Could you check a few things on this model? Use its own coordinates, in mm. A direction names the side the tool comes from. Round coordinates to 2 decimals unless told otherwise and drop trailing zeros. Loops run counter-clockwise (first coordinate to the right, second up) from the corner with the lowest first, then second, coordinate; pieces in that order, holes last. Notation, with made-up numbers: (71, -10) -> (124, -10) arc R18 ccw to (124, 10) -> close; hole circle Ø8 at (-40, -31). An arc over 180 degrees is marked (long way). One line per item, written item: value.
Autodesk Inventor part; units mm, degrees
ref_plane "YZ Plane" through (0, 0, 0) normal (1, 0, 0) x (0, 1, 0)
ref_plane "XZ Plane" through (0, 0, 0) normal (0, 1, 0) x (-1, 0, 0)
ref_plane "XY Plane" through (0, 0, 0) normal (0, 0, 1) x (1, 0, 0)
sketch "Sketch1" plane through (0, 0, 0) normal (0, 0, 1) x (1, 0, 0)
  line L0 (7.62, 0) -> (72.898, 0)
  line L1 (0, 7.62) -> (0, 31.242)
  line L2 (7.62, 38.862) -> (72.898, 38.862)
  line L3 (80.518, 31.242) -> (80.518, 7.62)
  arc A0 (7.62, 38.862) -> (0, 31.242) centre (7.62, 31.242) ccw
  arc A1 (80.518, 31.242) -> (72.898, 38.862) centre (72.898, 31.242) ccw
  arc A2 (72.898, 0) -> (80.518, 7.62) centre (72.898, 7.62) ccw
  arc A3 (0, 7.62) -> (7.62, 0) centre (7.62, 7.62) ccw
  point P0 (0, 0)
  point P1 (80.518, 0)
  point P2 (0, 38.862)
  dimension "d2" = 80.518
  dimension "d3" = 38.862
  dimension "d4" = 7.62
  dimension "d5" = 7.62
  dimension "d6" = 7.62
  dimension "d7" = 7.62
extrude "Extrusion1" add sketch "Sketch1" along normal blind 80.518
sketch "Sketch2" plane through (0, 0, 80.518) normal (0, 0, 1) x (1, 0, 0)
  line L0 (14.732, 7.62) -> (65.532, 7.62)
  line L1 (70.612, 12.7) -> (70.612, 26.162)
  line L2 (65.532, 31.242) -> (14.732, 31.242)
  line L3 (9.652, 26.162) -> (9.652, 12.7)
  arc A0 (14.732, 31.242) -> (9.652, 26.162) centre (14.732, 26.162) ccw
  arc A1 (70.612, 26.162) -> (65.532, 31.242) centre (65.532, 26.162) ccw
  arc A2 (65.532, 7.62) -> (70.612, 12.7) centre (65.532, 12.7) ccw
  arc A3 (9.652, 12.7) -> (14.732, 7.62) centre (14.732, 12.7) ccw
  point P0 (0, 0)
  point P1 (9.652, 7.62)
  point P2 (70.612, 7.62)
  point P3 (70.612, 31.242)
  dimension "d12" = 60.96
  dimension "d13" = 23.622
  dimension "d16" = 5.08
extrude "Extrusion2" cut sketch "Sketch2" against normal blind 14.478
sketch "Sketch3" plane through (7.62, 38.862, 0) normal (0, 1, 0) x (1, 0, 0)
  line L0 (60.198, -54.2068) -> (60.198, -23.9808)
  line L1 (55.118, -18.9008) -> (14.986, -18.9008)
  line L2 (9.906, -23.9808) -> (9.906, -54.2068)
  line L3 (14.986, -59.2868) -> (55.118, -59.2868)
  line L4 (72.898, 0) -> (72.898, -80.518)
  arc A0 (14.986, -18.9008) -> (9.906, -23.9808) centre (14.986, -23.9808) ccw
  arc A1 (60.198, -23.9808) -> (55.118, -18.9008) centre (55.118, -23.9808) ccw
  arc A2 (55.118, -59.2868) -> (60.198, -54.2068) centre (55.118, -54.2068) ccw
  arc A3 (9.906, -54.2068) -> (14.986, -59.2868) centre (14.986, -54.2068) ccw
  point P0 (-7.62, 0)
  point P1 (60.198, -59.2868)
  point P2 (60.198, -18.9008)
  point P3 (9.906, -18.9008)
  point P4 (9.906, -59.2868)
  dimension "d19" = 40.386
  dimension "d20" = 50.292
  dimension "d21" = 12.7
  dimension "d33" = 5.08
extrude "Extrusion3" cut sketch "Sketch3" against normal blind 27.178
sketch "Sketch4" plane through (0, 0, 0) normal (0, 0, -1) x (-1, 0, 0)
  line L0 (-8.6279, 26.924) -> (-8.6279, 11.684)
  line L1 (-72.1279, 11.684) -> (-72.1279, 26.924)
  line L2 (-67.0479, 32.004) -> (-13.7079, 32.004)
  line L3 (-13.7079, 6.604) -> (-67.0479, 6.604)
  arc A0 (-67.0479, 32.004) -> (-72.1279, 26.924) centre (-67.0479, 26.924) ccw
  arc A1 (-8.6279, 26.924) -> (-13.7079, 32.004) centre (-13.7079, 26.924) ccw
  arc A2 (-13.7079, 6.604) -> (-8.6279, 11.684) centre (-13.7079, 11.684) ccw
  arc A3 (-72.1279, 11.684) -> (-67.0479, 6.604) centre (-67.0479, 11.684) ccw
  point P0 (0, 0)
  point P1 (-8.6279, 32.004)
  point P2 (-8.6279, 6.604)
  point P3 (-72.1279, 6.604)
  point P4 (-72.1279, 32.004)
  dimension "d26" = 25.4
  dimension "d27" = 63.5
  dimension "d29" = 25.4
  dimension "d30" = 5.08
extrude "Extrusion4" cut sketch "Sketch4" against normal blind 14.478
sketch "Sketch5" plane through (80.518, 7.62, 0) normal (1, 0, 0) x (0, 0, -1)
  line L0 (-80.518, 23.622) -> (0, 23.622)
  line L1 (0, 23.622) -> (-80.518, 23.622)
  line L2 (0, 23.622) -> (0, 22.098)
  line L3 (0, 22.098) -> (-80.518, 22.098)
  line L4 (-80.518, 23.622) -> (-66.04, 23.622)
  line L5 (-80.518, 22.098) -> (-80.518, 23.622)
  line L6 (-80.518, 23.622) -> (-80.518, 22.098)
  point P0 (0, -7.62)
  dimension "d34" = 1.524
extrude "Extrusion5" cut sketch "Sketch5" against normal blind 1.27
sketch "Sketch6" plane through (0, 7.62, 0) normal (-1, 0, 0) x (0, 0, 1)
  line L0 (0, 23.622) -> (0, 22.098)
  line L1 (0, 23.622) -> (80.518, 23.622)
  line L2 (0, 22.098) -> (80.518, 22.098)
  line L3 (80.518, 23.622) -> (80.518, 22.098)
  line L4 (80.518, 22.098) -> (0, 22.098)
  line L5 (0, 22.098) -> (0, 23.622)
  point P0 (0, -7.62)
extrude "Extrusion6" cut sketch "Sketch6" against normal blind 1.27
properties part number "Body EM'" material "Wood (Birch)"
(1) Please list where these lines run through material, in increasing order: L1, parallel to Y at x = 26, z = 14; L2, parallel to Z at x = 48.5, y = 35.5; L3, parallel to Z at x = 38, y = 23.5.
Results below:
L1: y = 0 to 6.6, 32 to 38.86
L2: z = 0 to 18.9, 59.29 to 80.52
L3: z = 14.48 to 18.9, 59.29 to 66.04
(2) For pin 1 Ø3 at (x, y) = (18, 20) entering from -Z; pin 2 Ø1.4 at (x, z) = (1, 48.5) entering from -Y; pin 3 Ø1.5 at (x, z) = (48.5, 54) entering from +Y, each with a flat end and sliding along its axis, tell me the tip position at first contact or that it passes through.
Results below:
pin 1: stops at z = 14.48
pin 2: stops at y = 2.82
pin 3: stops at y = 11.68
(3) Imagine slicing it at C-C on z = 5.5. Write out the boundary of the cut face in (x, y), then the cut area to 3 significant figures.
Results below:
outline: (0, 7.62) arc R7.62 ccw to (7.62, 0) -> (72.9, 0) arc R7.62 ccw to (80.52, 7.62) -> (80.52, 29.72) -> (79.25, 29.72) -> (79.25, 31.24) -> (80.52, 31.24) arc R7.62 ccw to (72.9, 38.86) -> (7.62, 38.86) arc R7.62 ccw to (0, 31.24) -> (1.27, 31.24) -> (1.27, 29.72) -> (0, 29.72) -> close; hole (8.63, 11.68) arc R5.08 ccw to (13.71, 6.6) -> (67.05, 6.6) arc R5.08 ccw to (72.13, 11.68) -> (72.13, 26.92) arc R5.08 ccw to (67.05, 32) -> (13.71, 32) arc R5.08 ccw to (8.63, 26.92) -> close
area: 1,480 mm²
(4) Imagine slicing it at B-B on y = 17.5. Write out the boundary of the cut face in (x, z), then the cut area to 3 significant figures.
Results below:
outline: (0, 0) -> (8.63, 0) -> (8.63, 14.48) -> (72.13, 14.48) -> (72.13, 0) -> (80.52, 0) -> (80.52, 80.52) -> (70.61, 80.52) -> (70.61, 66.04) -> (9.65, 66.04) -> (9.65, 80.52) -> (0, 80.52) -> close; hole (17.53, 23.98) arc R5.08 ccw to (22.61, 18.9) -> (62.74, 18.9) arc R5.08 ccw to (67.82, 23.98) -> (67.82, 54.21) arc R5.08 ccw to (62.74, 59.29) -> (22.61, 59.29) arc R5.08 ccw to (17.53, 54.21) -> close
area: 2,670 mm²
(5) Imagine slicing it at A-A on x = 38.5. Write out the boundary of the cut face in (y, z).
Results below:
outline: (0, 0) -> (6.6, 0) -> (6.6, 14.48) -> (32, 14.48) -> (32, 0) -> (38.86, 0) -> (38.86, 18.9) -> (11.68, 18.9) -> (11.68, 59.29) -> (38.86, 59.29) -> (38.86, 80.52) -> (31.24, 80.52) -> (31.24, 66.04) -> (7.62, 66.04) -> (7.62, 80.52) -> (0, 80.52) -> close
(6) On a 3-axis mill with a long thin cutter (end or side, diameter ignored), from which of +Z, -Z, +X, -X, +Y, -Y can I reach the whole of each face in a straight line? I mean faces 1 (the face through (43, 25, 18.901)), 2 (the face through (0, 19, 40)), 3 (the face through (69.163, 29.714, 73.38)), 4 (the face through (70.6, 30.555, 7.138)). Say none if no direction works.
Results below:
face 1: +Y
face 2: +Z, -Z, -X, +Y, -Y
face 3: +Z
face 4: -Z
(7) We'd pull the mould along X, two halves only. Please class faces 5 (the face through (78.345, 2.291, 39.695)), 6 (the face through (40, 33, 0)), 7 (the face through (2.291, 2.173, 39.695)), 8 (the face through (42, 25, 59.287)): +X half, -X half, draft (parallel to the pull), parting line (faces both ways), or undercut.
Results below:
face 5: +X half
face 6: draft
face 7: -X half
face 8: undercut
(8) Imagine slicing it at D-D on z = 34.5. Write out the boundary of the cut face in (x, y).
Results below:
outline: (0, 7.62) arc R7.62 ccw to (7.62, 0) -> (72.9, 0) arc R7.62 ccw to (80.52, 7.62) -> (80.52, 29.72) -> (79.25, 29.72) -> (79.25, 31.24) -> (80.52, 31.24) arc R7.62 ccw to (72.9, 38.86) -> (67.82, 38.86) -> (67.82, 11.68) -> (17.53, 11.68) -> (17.53, 38.86) -> (7.62, 38.86) arc R7.62 ccw to (0, 31.24) -> (1.27, 31.24) -> (1.27, 29.72) -> (0, 29.72) -> close
